```python
from build123d import *

# Parameters (mm, degrees)
BOSS_EXTRUDE1_DEPTH  = 15
SKETCH8_W            = 10
SKETCH8_H            = 5.5
BOSS_EXTRUDE2_DEPTH  = 6
BOSS_EXTRUDE3_DEPTH  = 120
SKETCH10_W           = 8
SKETCH10_H           = 5.5
BOSS_EXTRUDE4_DEPTH  = 5
SKETCH11_W           = 5.5
SKETCH11_H           = 11.334625819
BOSS_EXTRUDE5_DEPTH  = 15
SKETCH12_W           = 10
SKETCH12_H           = 5.5
BOSS_EXTRUDE6_DEPTH  = 6
BOSS_EXTRUDE7_DEPTH  = 120
SKETCH14_W           = 9
SKETCH14_H           = 5.5
BOSS_EXTRUDE8_DEPTH  = 6
SKETCH15_W           = 104
SKETCH15_H           = 3
BOSS_EXTRUDE11_DEPTH = 8.5
CUT_EXTRUDE1_DEPTH   = 1.5


with BuildPart() as part:
    # Sketch2 → Boss-Extrude1 (new body)
    with BuildSketch(Plane(origin=(0, 0, 0), x_dir=(1, 0, 0), z_dir=(0, 1, 0))):
        Polygon((-98.263888889, -54.75), (-98.263888889, 59.75), (21.736111111, 59.75), (21.736111111, -54.75), (11.736111111, -54.75), (11.736111111, -60.25), (27.236111111, -60.25), (27.236111111, 65.25), (-103.763888889, 65.25), (-103.763888889, -60.25), (-3.263888889, -60.25), (-3.263888889, -54.75), align=None)
    extrude(amount=BOSS_EXTRUDE1_DEPTH)

    # Sketch8 → Boss-Extrude2 (add)
    with BuildSketch(Plane(origin=(0, 15, 0), x_dir=(1, 0, 0), z_dir=(0, 1, 0))):
        with Locations((-94.263888889, -57.5)):
            Rectangle(SKETCH8_W, SKETCH8_H)
    extrude(amount=BOSS_EXTRUDE2_DEPTH)

    # Sketch9 → Boss-Extrude3 (add)
    with BuildSketch(Plane(origin=(0, 0, 54.75), x_dir=(-1, 0, 0), z_dir=(0, 0, -1))):
        Polygon((90.263888889, 15), (90.263888889, 16), (90.263888889, 20), (98.263888889, 20), (98.263888889, 16), (98.263888889, 15), (99.263888889, 15), (99.263888889, 21), (89.263888889, 21), (89.263888889, 15), align=None)
    extrude(amount=BOSS_EXTRUDE3_DEPTH)

    # Sketch10 → Boss-Extrude4 (add)
    with BuildSketch(Plane(origin=(0, 15, 0), x_dir=(1, 0, 0), z_dir=(0, 1, 0))):
        with Locations((-94.263888889, 62.5)):
            Rectangle(SKETCH10_W, SKETCH10_H)
    extrude(amount=BOSS_EXTRUDE4_DEPTH)

    # Sketch11 → Boss-Extrude5 (add)
    with BuildSketch(Plane(origin=(-3.263888889, 0, 0), x_dir=(0, 0, -1), z_dir=(1, 0, 0))):
        with Locations((-57.5, 9.332687091)):
            Rectangle(SKETCH11_W, SKETCH11_H)
    extrude(amount=BOSS_EXTRUDE5_DEPTH)

    # Sketch12 → Boss-Extrude6 (add)
    with BuildSketch(Plane(origin=(0, 15, 0), x_dir=(1, 0, 0), z_dir=(0, 1, 0))):
        with Locations((17.736111111, -57.5)):
            Rectangle(SKETCH12_W, SKETCH12_H)
    extrude(amount=BOSS_EXTRUDE6_DEPTH)

    # Sketch13 → Boss-Extrude7 (add)
    with BuildSketch(Plane(origin=(0, 0, 54.75), x_dir=(-1, 0, 0), z_dir=(0, 0, -1))):
        Polygon((-21.736111111, 15), (-21.736111111, 16), (-21.736111111, 20), (-13.736111111, 20), (-13.736111111, 16), (-13.736111111, 15), (-12.736111111, 15), (-12.736111111, 21), (-22.736111111, 21), (-22.736111111, 15), align=None)
    extrude(amount=BOSS_EXTRUDE7_DEPTH)

    # Sketch14 → Boss-Extrude8 (add)
    with BuildSketch(Plane(origin=(0, 15, 0), x_dir=(1, 0, 0), z_dir=(0, 1, 0))):
        with Locations((18.236111111, 62.5)):
            Rectangle(SKETCH14_W, SKETCH14_H)
    extrude(amount=BOSS_EXTRUDE8_DEPTH)

    # Sketch15 → Boss-Extrude11 (add)
    with BuildSketch(Plane(origin=(0, 0, 54.75), x_dir=(-1, 0, 0), z_dir=(0, 0, -1))):
        with Locations((38.263888889, 13.5)):
            Rectangle(SKETCH15_W, SKETCH15_H)
    extrude(amount=BOSS_EXTRUDE11_DEPTH)

    # Sketch17 → Cut-Extrude1 (cut)
    with BuildSketch(Plane.XY.offset(-59.75)):
        Polygon((-98.263888889, 0), (21.736111111, 0), (21.736111111, 20), (13.736111111, 20), (13.736111111, 15), (12.736111111, 15), (-89.263888889, 15), (-90.263888889, 15), (-90.263888889, 20), (-98.263888889, 20), align=None)
    extrude(amount=-CUT_EXTRUDE1_DEPTH, mode=Mode.SUBTRACT)


solid = part.part
```
Could you check a few things on this model? Use its own coordinates, in mm. A direction names the side the tool comes from. Round coordinates to 2 decimals unless told otherwise and drop trailing zeros. Loops run counter-clockwise (first coordinate to the right, second up) from the corner with the lowest first, then second, coordinate; pieces in that order, holes last.
Q1. I want a section at A-A (z = 5.5). Write out the boundary of the cut face in (x, y), and give its area (3 significant figures).
Q2. On a 3-axis mill with a long thin cutter (end or side, diameter ignored), from which of +Z, -Z, +X, -X, +Y, -Y can I reach the whole of each face in a straight line? I mean faces 4 (the flat face through (-102, 15, -3)), 5 (the flat face through (-98.264, 10, -2)), 6 (the flat face through (11.736, 2, 57)), 7 (the flat face through (-39, 15, -63)). Say none if no direction works.
Q3. Thinking about a two-plate mould opening in Z: for faces 1 (the flat face through (-99.264, 18, -2)), 2 (the flat face through (13.736, 17, -2)), 3 (the flat face through (-90.264, 17, -2)), which applies, pulls with the +Z half, pulls with the -Z half, needs draft (parallel to the pull), parting line crosses it, or undercut?
Q4. For P1, Ø3, axis at y = 19, z = 12, coming from the +X side; P2, Ø6, axis at x = -44, z = 44, coming from the -Y side; P3, Ø6, axis at x = 3.5, z = 58, coming from the -Y side, each with a flat end and sliding along its axis, tell me the tip position at first contact or that it passes through.
Q5. I want a section at B-B (y = 8.75). Write out the boundary of the cut face in (x, z), and give its area (3 significant figures).
Q6. Please list where these lines run through material, in increasing order: L1, parallel to X at y = 15.25, z = -27.5; L2, parallel to X at y = 1.75, z = 20.5; L3, parallel to Z at x = 6, y = 9.5.
Q7. I want a section at C-C (x = -71). Write out the boundary of the cut face in (y, z), and give its area (3 significant figures).
Q8. I want a section at D-D (z = 48.5). Write out the boundary of the cut face in (x, y), and give its area (3 significant figures).
Answer below:
1. outline: (-103.76, 0) - (-98.26, 0) - (-98.26, 20) - (-90.26, 20) - (-90.26, 15) - (-89.26, 15) - (-89.26, 21) - (-99.26, 21) - (-99.26, 15) - (-103.76, 15) - close; (12.74, 15) - (13.74, 15) - (13.74, 20) - (21.74, 20) - (21.74, 0) - (27.24, 0) - (27.24, 15) - (22.74, 15) - (22.74, 21) - (12.74, 21) - close
1. area: 205 mm2
2. face 4: +Z, -Z, -X, +Y
2. face 5: -Y
2. face 6: +Z, -Y
2. face 7: +Z, -Z, +Y
3. face 1: needs draft
3. face 2: undercut
3. face 3: undercut
4. P1: stops at x = 22.74
4. P2: stops at y = 12
4. P3: stops at y = 3.67
5. outline: (-103.76, -65.25) - (27.24, -65.25) - (27.24, 60.25) - (-103.76, 60.25) - close; hole (-98.26, -61.25) - (21.74, -61.25) - (21.74, 54.75) - (-98.26, 54.75) - close
5. area: 2,520 mm2
6. L1: x = -99.26 to -98.26, -90.26 to -89.26, 12.74 to 13.74, 21.74 to 22.74
6. L2: x = -103.76 to -98.26, 21.74 to 27.24
6. L3: z = -65.25 to -61.25, 54.75 to 60.25
7. outline: (0, -65.25) - (15, -65.25) - (15, -61.25) - (0, -61.25) - close; (0, 54.75) - (12, 54.75) - (12, 46.25) - (15, 46.25) - (15, 60.25) - (0, 60.25) - close
7. area: 168 mm2
8. outline: (-103.76, 0) - (-98.26, 0) - (-98.26, 20) - (-90.26, 20) - (-90.26, 12) - (13.74, 12) - (13.74, 20) - (21.74, 20) - (21.74, 0) - (27.24, 0) - (27.24, 15) - (22.74, 15) - (22.74, 21) - (12.74, 21) - (12.74, 15) - (-89.26, 15) - (-89.26, 21) - (-99.26, 21) - (-99.26, 15) - (-103.76, 15) - close
8. area: 517 mm2
